Geometry: final body of the model. Coordinates: model frame, mm. Face numbers are marked on the shaded views. A direction names the side the tool comes from. Give positions to 0.01 mm unless a question says otherwise; leave off trailing zeros. Write each loop counter-clockwise with the first axis right and the second up, starting at its lowest first coordinate (ties: lowest second). Pieces come first, ordered by that corner, then holes.
Q1. Pin query (flat end, axial travel): pin 1 (1.5 mm diameter, centred on x = -16.5, z = 2.5, fed in from -Y) (3 decimals); pin 2 (10 mm diameter, centred on x = 17.5, z = -3.5, fed in from +Y); pin 3 (9.5 mm diameter, centred on x = 3.5, y = 2.5, fed in from -Z); pin 4 (5 mm diameter, centred on x = 2.5, z = 3, fed in from -Y). Return the tip coordinate at first contact, or that it passes through.
Q2. Cut plane C-C on x = 7. Return the cut outline in (y, z) (3 decimals), plus the area to 3 significant figures.
Q3. Line query: L1, parallel to Y at x = 0, z = 10.3 (3 decimals); L2, parallel to X at y = -2, z = 3.5; L3, parallel to Z at x = -20, y = -4. Output: solid intervals per line, ascending.
Q4. Reachability of the marked faces 4, 5, 6 and 7 from +Z, -Z, +X, -X, +Y, -Y: full face, straight path, thin tool, end or side. Return the list, or none.
Q5. Draft query along Z for the marked faces 1, 2 and 3. Return one class per face: pulls with the +Z half, pulls with the -Z half, needs draft (parallel to the pull), parting line crosses it, or undercut.
Q6. Cut plane B-B on z = 11.75. Return the cut outline in (x, y) (3 decimals), plus the area to 3 significant figures.
Q7. Cut plane D-D on x = -4. Return the cut outline in (y, z) (3 decimals), plus the area to 3 significant figures.
Q8. Cut plane A-A on z = 0. Count the separate pieces of the cut face and the enclosed holes in it, plus the area to 3 significant figures.
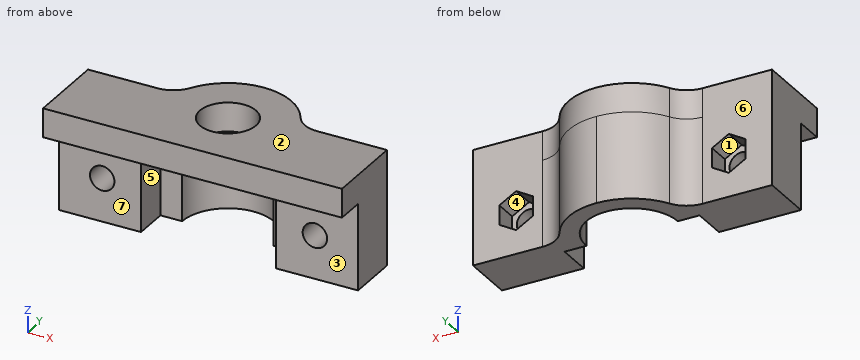
```python
from build123d import *

# Parameters (mm, degrees)
F0_R      = 4.75
F1_DEPTH  = 7.5
F2_R      = 2.125
F3_DEPTH  = 25
F5_DEPTH  = 15.001
F7_DEPTH  = 7.5
F8_R      = 4.875
F9_DEPTH  = 5
F10_W     = 51.95911
F10_H     = 5
F11_DEPTH = 5
F12_W     = 11.8
F12_H     = 20
F13_DEPTH = 4
F14_R     = 5
F16_DEPTH = 25


with BuildPart() as f1:
    # F0 (on Top) → F1 (new body, symmetric)
    with BuildSketch(Plane.XY):
        with BuildLine():
            Line((-10.979555, -11.025), (0, -11.025))
            Line((0, -11.025), (10.979555, -11.025))
            Line((10.979555, -11.025), (10.979555, -6.025))
            Line((10.979555, -6.025), (25.979555, -6.025))
            Line((25.979555, -6.025), (25.979555, -1.025))
            Line((25.979555, -1.025), (10.979555, -1.025))
            Line((10.979555, -1.025), (10.979555, 1))
            ThreePointArc((10.979555, 1), (7.433896, 8.141733), (0, 11.025))
            ThreePointArc((0, 11.025), (-7.433896, 8.141733), (-10.979555, 1))
            Line((-10.979555, 1), (-10.979555, -1.025))
            Line((-10.979555, -1.025), (-25.979555, -1.025))
            Line((-25.979555, -1.025), (-25.979555, -6.025))
            Line((-25.979555, -6.025), (-10.979555, -6.025))
            Line((-10.979555, -6.025), (-10.979555, -11.025))
        make_face()
        Circle(F0_R, mode=Mode.SUBTRACT)
    extrude(amount=F1_DEPTH, both=True)

    # F2 (on face) → F3 (cut)
    with BuildSketch(Plane.XZ.offset(11.025)):
        with Locations((-18.479555, 0)):
            Circle(F2_R)
        with Locations((18.479555, 0)):
            Circle(F2_R)
    extrude(amount=-F3_DEPTH, mode=Mode.SUBTRACT)

    # F4 (on face) → F5 (cut, through all)
    with BuildSketch(Plane.XY.offset(7.5)):
        with BuildLine():
            Line((10.979555, -0.0125), (7.82499, -0.0125))
            ThreePointArc((7.82499, -0.0125), (0, 7.825), (-7.82499, -0.0125))
            Line((-7.82499, -0.0125), (-10.979555, -0.0125))
            Line((-10.979555, -0.0125), (-10.979555, -6.025))
            Line((-10.979555, -6.025), (-10.979555, -11.025))
            Line((-10.979555, -11.025), (10.979555, -11.025))
            Line((10.979555, -11.025), (10.979555, -6.025))
            Line((10.979555, -6.025), (10.979555, -0.0125))
        make_face()
    extrude(amount=-F5_DEPTH, mode=Mode.SUBTRACT)

    # F6 (on Top) → F7 (join, symmetric)
    with BuildSketch(Plane.XY):
        with BuildLine():
            Line((-10.979555, -1.025), (-10.979555, 1))
            ThreePointArc((-10.979555, 1), (-10.842852, 1.995794), (-10.616026, 2.975))
            Line((-10.616026, 2.975), (-14.179555, 2.975))
            Line((-14.179555, 2.975), (-14.179555, -1.025))
            Line((-14.179555, -1.025), (-10.979555, -1.025))
        make_face()
        with BuildLine():
            Line((14.179555, 2.975), (10.616026, 2.975))
            ThreePointArc((10.616026, 2.975), (10.842852, 1.995794), (10.979555, 1))
            Line((10.979555, 1), (10.979555, -1.025))
            Line((10.979555, -1.025), (14.179555, -1.025))
            Line((14.179555, -1.025), (14.179555, 2.975))
        make_face()
    extrude(amount=F7_DEPTH, both=True)

    # F8 (on face) → F9 (join)
    with BuildSketch(Plane.XY.offset(7.5)):
        with BuildLine():
            Line((-25.979555, -6.025), (-10.979555, -6.025))
            Line((-10.979555, -6.025), (10.979555, -6.025))
            Line((10.979555, -6.025), (25.979555, -6.025))
            Line((25.979555, -6.025), (25.979555, -1.025))
            Line((25.979555, -1.025), (14.179555, -1.025))
            Line((14.179555, -1.025), (14.179555, 2.975))
            Line((14.179555, 2.975), (10.616026, 2.975))
            ThreePointArc((10.616026, 2.975), (0, 11.025), (-10.616026, 2.975))
            Line((-10.616026, 2.975), (-14.179555, 2.975))
            Line((-14.179555, 2.975), (-14.179555, -1.025))
            Line((-14.179555, -1.025), (-25.979555, -1.025))
            Line((-25.979555, -1.025), (-25.979555, -6.025))
        make_face()
        Circle(F8_R, mode=Mode.SUBTRACT)
    extrude(amount=F9_DEPTH)

    # F10 (on face) → F11 (join)
    with BuildSketch(Plane.XZ.offset(6.025)):
        with Locations((0, 10)):
            Rectangle(F10_W, F10_H)
    extrude(amount=F11_DEPTH)

    # F12 (on face) → F13 (join)
    with BuildSketch(Plane(origin=(0, -1.025, 0), x_dir=(-1, 0, 0), z_dir=(0, 1, 0))):
        with Locations((-20.079555, 2.5)):
            Rectangle(F12_W, F12_H)
        Polygon((-18.479555, 3.377499), (-15.554555, 1.68875), (-15.554555, -1.68875), (-18.479555, -3.377499), (-21.404555, -1.68875), (-21.404555, 1.68875), align=None, mode=Mode.SUBTRACT)
        with Locations((20.079555, 2.5)):
            Rectangle(F12_W, F12_H)
        Polygon((15.554555, 1.68875), (18.479555, 3.377499), (21.404555, 1.68875), (21.404555, -1.68875), (18.479555, -3.377499), (15.554555, -1.68875), align=None, mode=Mode.SUBTRACT)
    extrude(amount=F13_DEPTH)

    # F14
    f14_edges = [f1.edges().sort_by_distance(p)[0] for p in [
        (6.661503, 8.78493, 0),
        (10.616026, 2.975, 10),
        (-6.661503, 8.78493, 0),
        (-10.616026, 2.975, 10),
    ]]
    fillet(f14_edges, radius=F14_R)

    # F15 (on face) → F16 (cut)
    with BuildSketch(Plane(origin=(0, 0, 7.5), x_dir=(1, 0, 0), z_dir=(0, 0, -1))):
        with BuildLine():
            Line((11.729555, 6.025), (-11.729555, 6.025))
            Line((-11.729555, 6.025), (-11.729555, 0))
            Line((-11.729555, 0), (-7.95, 0))
            ThreePointArc((-7.95, 0), (0, -7.95), (7.95, 0))
            Line((7.95, 0), (11.729555, 0))
            Line((11.729555, 0), (11.729555, 6.025))
        make_face()
    extrude(amount=F16_DEPTH, mode=Mode.SUBTRACT)


solid = f1.part
```
Data:
1. pin 1: stops at y = -6.025
1. pin 2: stops at y = 3.17
1. pin 3: stops at z = -7.5
1. pin 4: stops at y = 6.18
2. outline: (-11.025, 7.5) - (3.769, 7.5) - (3.769, -7.5) - (8.518, -7.5) - (8.518, 12.5) - (-11.025, 12.5) - close
2. area: 169 mm2
3. L1: y = -11.025 to -4.875, 4.875 to 11.025
3. L2: x = -25.98 to -11.73, 11.73 to 25.98
3. L3: z = -7.5 to -1.48, 1.48 to 12.5
4. face 4: +Y
4. face 5: -Z, -Y
4. face 6: +Z, -Z, -X, +Y
4. face 7: -Z, +X, -X, -Y
5. face 1: undercut
5. face 2: pulls with the +Z half
5. face 3: needs draft
6. outline: (-25.98, -11.025) - (25.98, -11.025) - (25.98, 2.975) - (13.9, 2.975) arc R5 cw to (9.563, 5.487) arc R11.025 ccw to (-9.563, 5.487) arc R5 cw to (-13.9, 2.975) - (-25.98, 2.975) - close; hole circle Ø9.75 at (0, 0)
6. area: 782 mm2
7. outline: (-11.025, 7.5) - (-2.787, 7.5) - (-2.787, 12.5) - (-11.025, 12.5) - close; (2.787, 7.5) - (6.87, 7.5) - (6.87, -7.5) - (10.274, -7.5) - (10.274, 12.5) - (2.787, 12.5) - close
7. area: 130 mm2
8. separate pieces: 3
8. enclosed holes: 0
8. area: 267 mm2
